Answer from the drawing. Dimensions are ordinates in mm from the lowest x, y and z of the part. A direction names the side the tool comes from. Coordinates: 2 decimals unless noted, no trailing zeros. Order: outer loops, then holes, each group sorted by start corner. A loop starts at its lowest first (then second) coordinate and runs counter-clockwise, first axis right, second up. Notation, with made-up numbers: (8, 74) -> (26, 74) arc R23 ccw to (26, 98) -> close; hole circle Ø9 at (57, 54). An arc over 180 degrees is marked (long way). Answer in a Markdown table with one row per item.
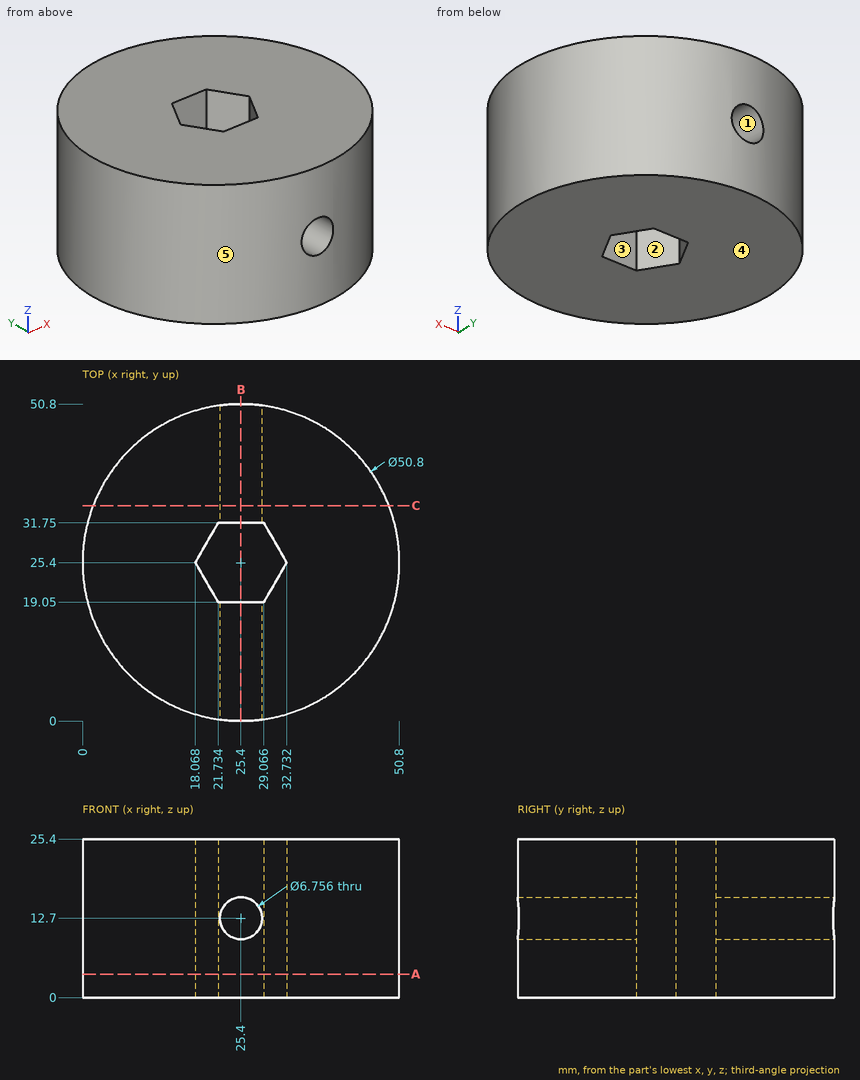
(1) A cutting plane is placed at C-C, the plane y = 34.5. Determine the outline of the cut face in (x, z), then the cut area to 3 significant figures.
Check values:
| item | result |
|---|---|
| outline | (1.69, 0) -> (49.11, 0) -> (49.11, 25.4) -> (1.69, 25.4) -> close; hole circle Ø6.76 at (25.4, 12.7) |
| area | 1,170 mm² |
(2) Flat-ended cylindrical pins translate along their axes: pin 1 (6 mm diameter, centred on x = 32.5, z = 21.5, fed in from -Y); pin 2 (4 mm diameter, centred on x = 13, z = 21, fed in from -Y); pin 3 (10 mm diameter, centred on y = 7, z = 17.5, fed in from -X); pin 4 (8 mm diameter, centred on x = 25.4, z = 12.7, fed in from -Y). Find the tip coordinate at first contact, or state that the pin passes through.
Check values:
| item | result |
|---|---|
| pin 1 | y = 0.33 |
| pin 2 | y = 2.23 |
| pin 3 | x = 3.82 |
| pin 4 | y = 0 |
(3) Find the intervals of material crossed by line 1 along Z through (x, y) = (25.5, 42); line 2 along X through (y, z) = (30, 15.5) (1 decimal); line 3 along Y through (x, z) = (26, 8.5), in increasing order. Write a range as from..to.
Check values:
| item | result |
|---|---|
| line 1 | 0..9.32, 16.08..25.4 |
| line 2 | 0.4..20.7, 30.1..50.4 |
| line 3 | 0.01..19.05, 31.75..50.79 |
(4) For a pull along X with two mould halves and no side action, classify the marked faces 3, 4 and 5 as released by +X, released by -X, zero draft, split by the parting line, or undercut.
Check values:
| item | result |
|---|---|
| face 3 | undercut |
| face 4 | zero draft |
| face 5 | split by the parting line |
(5) Which of the six approach directions +Z, -Z, +X, -X, +Y, -Y give full straight-line access (tool end or side, diameter ignored) to the marked faces 1 and 2?
Check values:
| item | result |
|---|---|
| face 1 | +Y, -Y |
| face 2 | +Z, -Z |
(6) A cutting plane is placed at A-A, the plane z = 3.75. Determine the outline of the cut face in (x, y).
Check values:
| item | result |
|---|---|
| outline | circle Ø50.8 at (25.4, 25.4); hole (18.07, 25.4) -> (21.73, 19.05) -> (29.07, 19.05) -> (32.73, 25.4) -> (29.07, 31.75) -> (21.73, 31.75) -> close |
(7) A cutting plane is placed at B-B, the plane x = 25.4. Determine the outline of the cut face in (y, z).
Check values:
| item | result |
|---|---|
| outline | (0, 0) -> (19.05, 0) -> (19.05, 9.32) -> (0, 9.32) -> close; (0, 16.08) -> (19.05, 16.08) -> (19.05, 25.4) -> (0, 25.4) -> close; (31.75, 0) -> (50.8, 0) -> (50.8, 9.32) -> (31.75, 9.32) -> close; (31.75, 16.08) -> (50.8, 16.08) -> (50.8, 25.4) -> (31.75, 25.4) -> close |
